```python
from build123d import *

# Parameters (mm, degrees)
SKETCH1_W                 = 30
SKETCH1_H                 = 30
BOSS_EXTRUDE1_DEPTH       = 80
SKETCH2_R                 = 6
BOSS_EXTRUDE2_DEPTH       = 20
CUT_EXTRUDE1_DEPTH        = 83.764726786
BOSS_EXTRUDE3_DEPTH       = 65
BOSS_EXTRUDE5_DEPTH       = 2
BOSS_EXTRUDE6_DEPTH       = 23
BOSS_EXTRUDE7_DEPTH       = 25
FILLET1_R                 = 2
SKETCH11_R                = 6.055782361
CUT_EXTRUDE2_DEPTH        = 2.125
CUT_EXTRUDE4_DEPTH        = 274.267856233
CUT_EXTRUDE4_DEPTH_BACK   = 274.267856233
SKETCH13_W                = 13.25
SKETCH13_H                = 8.5
FILLET2_R                 = 2
CUT_EXTRUDE6_REACH        = 234.702
SKETCH16_W                = 3.75
SKETCH16_H                = 3.75
FILLET4_R                 = 1
BOSS_EXTRUDE8_REACH       = 264.25
SKETCH17_W                = 22
SKETCH17_H                = 20
SKETCH18_W                = 17
SKETCH18_H                = 15
CUT_EXTRUDE7_DEPTH        = 66
FILLET5_R                 = 2
FILLET6_R                 = 2
CHAMFER1_SIZE             = 7
BOSS_EXTRUDE9_DEPTH       = 30
BOSS_EXTRUDE10_DEPTH      = 8
BOSS_EXTRUDE10_DEPTH_BACK = 8


with BuildPart() as part:
    # Sketch1 → Boss-Extrude1 (new body)
    with BuildSketch(Plane(origin=(0, 0, 0), x_dir=(1, 0, 0), z_dir=(0, 1, 0))):
        Rectangle(SKETCH1_W, SKETCH1_H)
    extrude(amount=BOSS_EXTRUDE1_DEPTH)

    # Sketch2 → Boss-Extrude2 (add)
    with BuildSketch(Plane(origin=(0, 80, 0), x_dir=(1, 0, 0), z_dir=(0, 1, 0))):
        with Locations(Location((9, -9, 0), (0, 0, 270))):
            Circle(SKETCH2_R)
    extrude(amount=BOSS_EXTRUDE2_DEPTH)

    # Sketch3 → Cut-Extrude1 (cut, through all)
    with BuildSketch(Plane(origin=(0, 80, 0), x_dir=(1, 0, 0), z_dir=(0, 1, 0))):
        with BuildLine():
            Line((9, -15), (15, -15))
            Line((15, -15), (15, -9))
            ThreePointArc((15, -9), (13.242640687, -13.242640687), (9, -15))
        make_face()
    extrude(amount=-CUT_EXTRUDE1_DEPTH, mode=Mode.SUBTRACT)

    # Sketch4 → Boss-Extrude3 (add)
    with BuildSketch(Plane(origin=(0, 80, 0), x_dir=(1, 0, 0), z_dir=(0, 1, 0))):
        Polygon((-11.25, 1.75), (-1.75, 1.75), (-1.75, 11.25), (-1.75, 15), (1.25, 15), (1.25, 11.25), (1.25, -1.25), (-11.25, -1.25), (-15, -1.25), (-15, 1.75), align=None)
        Polygon((-11.25, 8.25), (-8.25, 8.25), (-8.25, 11.25), (-8.25, 15), (-11.25, 15), (-11.25, 11.25), (-15, 11.25), (-15, 8.25), align=None)
    extrude(amount=BOSS_EXTRUDE3_DEPTH)

    # Sketch6 → Boss-Extrude5 (add)
    with BuildSketch(Plane.XZ):
        with BuildLine():
            Line((15, -15), (7, -15))
            Line((7, -15), (7, -177.175))
            ThreePointArc((7, -177.175), (2.757359313, -187.417640687), (13, -183.175))
            Line((13, -183.175), (15, -183.175))
            Line((15, -183.175), (15, -15))
        make_face()
    extrude(amount=-BOSS_EXTRUDE5_DEPTH)

    # Sketch7 → Boss-Extrude6 (add)
    with BuildSketch(Plane(origin=(0, 2, 0), x_dir=(1, 0, 0), z_dir=(0, 1, 0))):
        with BuildLine():
            Line((9, 188.831854249), (9, 186.639101615))
            ThreePointArc((9, 186.639101615), (7, 179.175), (5, 186.639101615))
            Line((5, 186.639101615), (5, 188.831854249))
            ThreePointArc((5, 188.831854249), (1.086408642, 182.160388128), (7, 177.175))
            Line((7, 177.175), (7, 15))
            Line((7, 15), (15, 15))
            Line((15, 15), (15, 183.175))
            Line((15, 183.175), (13, 183.175))
            ThreePointArc((13, 183.175), (11.898979486, 186.639101615), (9, 188.831854249))
        make_face()
    extrude(amount=BOSS_EXTRUDE6_DEPTH)

    # Sketch9 → Boss-Extrude7 (add)
    with BuildSketch(Plane.XZ):
        with BuildLine():
            Line((-15, 15), (-15, 7))
            Line((-15, 7), (-99.5, 7))
            ThreePointArc((-99.5, 7), (-99.577697751, 6.037536458), (-99.80877869, 5.1))
            Line((-99.80877869, 5.1), (-102.122778509, 5.1))
            ThreePointArc((-102.122778509, 5.1), (-109.375, 7), (-102.122778509, 8.9))
            Line((-102.122778509, 8.9), (-99.625, 8.9))
            ThreePointArc((-99.625, 8.9), (-101.816885554, 11.955834237), (-105.375001601, 13.173329766))
            Line((-105.375001601, 13.173329766), (-105.375001601, 15))
            Line((-105.375001601, 15), (-15, 15))
        make_face()
    extrude(amount=-BOSS_EXTRUDE7_DEPTH)

    # Fillet1
    fillet1_edges = [part.edges().sort_by_distance(p)[0] for p in [
        (-99.5, 12.5, 7),
    ]]
    fillet(fillet1_edges, radius=FILLET1_R)

    # Sketch11 → Cut-Extrude2 (cut)
    with BuildSketch(Plane.XZ):
        with Locations((-105.5, 7)):
            Circle(SKETCH11_R)
    extrude(amount=-CUT_EXTRUDE2_DEPTH, mode=Mode.SUBTRACT)

    # Sketch13 → Cut-Extrude4 (cut, two sides: drawn at the far end of the back side and taken through both)
    with BuildSketch(Plane.XY.offset(15).offset(-CUT_EXTRUDE4_DEPTH_BACK)):
        with Locations((-8.375, 72.75)):
            Rectangle(SKETCH13_W, SKETCH13_H)
    extrude(amount=CUT_EXTRUDE4_DEPTH + CUT_EXTRUDE4_DEPTH_BACK, mode=Mode.SUBTRACT)

    # Fillet2
    fillet2_edges = [part.edges().sort_by_distance(p)[0] for p in [
        (1.25, 112.5, 1.25),
    ]]
    fillet(fillet2_edges, radius=FILLET2_R)

    # Sketch16 → Cut-Extrude6 (cut, up to next)
    with BuildSketch(Plane(origin=(0, 80, 0), x_dir=(1, 0, 0), z_dir=(0, 1, 0)), mode=Mode.PRIVATE) as cut_extrude6_sk1:
        with Locations((-13.125, 13.125)):
            Rectangle(SKETCH16_W, SKETCH16_H)
    cut_extrude6_tool1 = extrude(cut_extrude6_sk1.sketch, amount=-CUT_EXTRUDE6_REACH, mode=Mode.PRIVATE) & part.part
    add(cut_extrude6_tool1.solids().sort_by_distance((-13.125, 80, -13.125))[0], mode=Mode.SUBTRACT)

    # Fillet4
    fillet4_edges = [part.edges().sort_by_distance(p)[0] for p in [
        (-11.25, 111, -11.25),
        (-15, 111, -11.25),
        (-11.25, 111, -15),
        (-15, 112.5, 1.25),
        (1.25, 112.5, -15),
    ]]
    fillet(fillet4_edges, radius=FILLET4_R)

    # Boss-Extrude8: up to this face of the body (flat: up to its plane)
    boss_extrude8_end = Plane(part.part.faces().sort_by_distance((-8.375, 68.5, 0))[0])
    # Sketch17 → Boss-Extrude8 (add, up to the picked face)
    with BuildSketch(Plane.XZ, mode=Mode.PRIVATE) as boss_extrude8_sk1:
        with Locations((-4, -126.63125)):
            Rectangle(SKETCH17_W, SKETCH17_H)
    boss_extrude8_tool1 = split(extrude(boss_extrude8_sk1.sketch, amount=-BOSS_EXTRUDE8_REACH, mode=Mode.PRIVATE), bisect_by=boss_extrude8_end, keep=Keep.BOTH, mode=Mode.PRIVATE)
    add(boss_extrude8_tool1.solids().sort_by(Axis((-4, 0, -126.63125), (0, 1, 0)))[0])

    # Sketch18 → Cut-Extrude7 (cut)
    with BuildSketch(Plane.XZ):
        with Locations((-4, -126.63125)):
            Rectangle(SKETCH18_W, SKETCH18_H)
    extrude(amount=-CUT_EXTRUDE7_DEPTH, mode=Mode.SUBTRACT)

    # Fillet5
    fillet5_edges = [part.edges().sort_by_distance(p)[0] for p in [
        (7, 12.5, -116.63125),
        (7, 12.5, -136.63125),
        (-15, 34.25, -136.63125),
        (-15, 34.25, -116.63125),
    ]]
    fillet(fillet5_edges, radius=FILLET5_R)

    # Fillet6
    fillet6_edges = [part.edges().sort_by_distance(p)[0] for p in [
        (7, 46.75, -116.63125),
        (7, 46.75, -136.63125),
    ]]
    fillet(fillet6_edges, radius=FILLET6_R)

    # Chamfer1
    chamfer1_edges = [part.edges().sort_by_distance(p)[0] for p in [
        (-12.5, 66, -126.63125),
        (-4, 66, -119.13125),
        (4.5, 66, -126.63125),
        (-4, 66, -134.13125),
    ]]
    chamfer(chamfer1_edges, length=CHAMFER1_SIZE)

    # Sketch19 → Boss-Extrude9 (add)
    with BuildSketch(Plane.XY.offset(15)):
        Polygon((-15, 51), (-25, 51), (-15, 41), align=None)
    extrude(amount=-BOSS_EXTRUDE9_DEPTH)

    # Sketch20 → Boss-Extrude10 (add, two sides: drawn at the far end of the back side and taken through both)
    with BuildSketch(Plane(origin=(0, 0, -126.63125), x_dir=(-1, 0, 0), z_dir=(0, 0, -1)).offset(-BOSS_EXTRUDE10_DEPTH_BACK)):
        Polygon((25, 51), (15, 51), (15, 41), align=None)
    extrude(amount=BOSS_EXTRUDE10_DEPTH + BOSS_EXTRUDE10_DEPTH_BACK)


solid = part.part
```
Read the model definition and answer for the solid it produces. Units are mm, in the model's axes. A direction names the side the tool comes from. Coordinates: 2 decimals unless noted, no trailing zeros. Order: outer loops, then holes, each group sorted by start corner. A loop starts at its lowest first (then second) coordinate and runs counter-clockwise, first axis right, second up. Notation, with made-up numbers: (-31, 14.25) - (9, 14.25) arc R26 ccw to (9, 40.25) - close; hole circle Ø7 at (85.25, 13.5). An arc over 180 degrees is marked (long way). Answer as a JSON object with one key per item and string values. Group by question number.
Item 1: Flat-ended cylindrical pins translate along their axes: P1, Ø0.9, axis at y = 121.5, z = -13, coming from the -X side; P2, Ø3.5, axis at x = -12.5, y = 103, coming from the +Z side; P3, Ø5, axis at y = 19.5, z = -25.5, coming from the -X side. Find the tip coordinate at first contact, or state that the pin passes through.
Item 2: Section C-C (y = 36.5) is taken. Give the vertices of the cut face in (x, z), plus the area to 3 significant figures.
Item 3: Consider probe 1 along Z at (x, y) = (-4, 21); probe 2 along Y at (x, z) = (-4, -7.5); probe 3 along Z at (x, y) = (2.5, 12). Determine where each line is inside the solid, lowest interval first. Write a range as from..to.
Item 4: Section B-B (y = 85) is taken. Give the vertices of the cut face in (x, z).
Item 5: A tool of negligible diameter and unlimited length cuts with its end or side. For faces 5 (the face through (-20, 46, 0)), 6 (the face through (-12.5, 29, -127)), 7 (the face through (-4, 68.5, -127)), from which of +Z, -Z, +X, -X, +Y, -Y can it reach the whole face along a straight path? Write none if from no direction.
Item 6: Section A-A (y = 129) is taken. Give the vertices of the cut face in (x, z), plus the area to 3 significant figures.
Item 7: The mould has two halves that part along Z. Classify faces 1 (the face through (-4, 29, -119.131)), 2 (the face through (-20, 51, 0)), 3 (the face through (4.5, 29, -127)), 4 (the face through (-7, 112, 1.25)): +Z half, -Z half, draft (parallel to the pull), parting line (faces both ways), or undercut.
Item 8: Section D-D (x = -51.5) is taken. Give the vertices of the cut face in (y, z).
Results are:
{
 "1": {"P1": "stops at x = -11.25", "P2": "stops at z = 1.25", "P3": "stops at x = 7"},
 "2": {"outline": "(-15, -134.63) arc R2 ccw to (-13, -136.63) - (5, -136.63) arc R2 ccw to (7, -134.63) - (7, -118.63) arc R2 ccw to (5, -116.63) - (-13, -116.63) arc R2 ccw to (-15, -118.63) - close; (-15, -15) - (15, -15) - (15, 9) arc R6 ccw to (9, 15) - (-15, 15) - close; hole (-12.5, -134.13) - (4.5, -134.13) - (4.5, -119.13) - (-12.5, -119.13) - close", "area": "1,070 mm^2"},
 "3": {"probe 1": "z = -136.63..-134.13, -119.13..-116.63, -15..15", "probe 2": "y = 0..68.5, 77..80", "probe 3": "z = -187.14..-179.21, -136.63..-134.13, -119.13..-116.63, -15..15"},
 "4": {"outline": "(-15, -10.25) arc R1 ccw to (-14, -11.25) - (-12.25, -11.25) arc R1 cw to (-11.25, -12.25) - (-11.25, -14) arc R1 ccw to (-10.25, -15) - (-8.25, -15) - (-8.25, -8.25) - (-15, -8.25) - close; (-15, -1.75) - (-1.75, -1.75) - (-1.75, -15) - (0.25, -15) arc R1 ccw to (1.25, -14) - (1.25, -0.75) arc R2 ccw to (-0.75, 1.25) - (-14, 1.25) arc R1 ccw to (-15, 0.25) - close; circle Ø12 at (9, 9)"},
 "5": {"face 5": "+Z, -Z, -X", "face 6": "-Y", "face 7": "-Z, +X, -X, +Y"},
 "6": {"outline": "(-15, -10.25) arc R1 ccw to (-14, -11.25) - (-12.25, -11.25) arc R1 cw to (-11.25, -12.25) - (-11.25, -14) arc R1 ccw to (-10.25, -15) - (-8.25, -15) - (-8.25, -8.25) - (-15, -8.25) - close; (-15, -1.75) - (-1.75, -1.75) - (-1.75, -15) - (0.25, -15) arc R1 ccw to (1.25, -14) - (1.25, -0.75) arc R2 ccw to (-0.75, 1.25) - (-14, 1.25) arc R1 ccw to (-15, 0.25) - close", "area": "118 mm^2"},
 "7": {"face 1": "undercut", "face 2": "draft", "face 3": "undercut", "face 4": "+Z half"},
 "8": {"outline": "(0, 7) - (25, 7) - (25, 15) - (0, 15) - close"}
}
